For this review, take the finished solid that the model builds, in its own axes (mm). Face numbers are marked on the shaded views. Round coordinates to 2 decimals unless told otherwise and drop trailing zeros. Write each loop counter-clockwise with the first axis right and the second up, starting at its lowest first coordinate (ties: lowest second). Pieces come first, ordered by that corner, then holes. Notation, with made-up numbers: (83.5, -14.5) -> (95.5, -14.5) arc R19 cw to (95.5, -2.5) -> close; hole circle Ø8 at (61, 13). An arc over 180 degrees is marked (long way). Write item = value, one per line. Start each with the question number.
```python
from build123d import *

# Parameters (mm, degrees)
F0_R     = 16.5
F0_R_2   = 14
F1_DEPTH = 125
F0_R_3   = 19
F2_DEPTH = 65
F3_DEPTH = 60
F4_SIZE  = 2.49999


# Not quite as in the source:
# - a fillet or chamfer is up to 0.001 mm smaller than in the source, because OpenCascade refuses the exact size


with BuildPart() as f1:
    # F0 (on Top) → F1 (new body)
    with BuildSketch(Plane.XY):
        Circle(F0_R)
        Circle(F0_R_2, mode=Mode.SUBTRACT)
    extrude(amount=F1_DEPTH)

    # F0 (on Top) → F2 (join)
    with BuildSketch(Plane.XY):
        Circle(F0_R_3)
        Circle(F0_R, mode=Mode.SUBTRACT)
    extrude(amount=F2_DEPTH)

    # F0 (on Top) → F3 (cut)
    with BuildSketch(Plane.XY):
        Circle(F0_R_3)
        Circle(F0_R, mode=Mode.SUBTRACT)
    extrude(amount=F3_DEPTH, mode=Mode.SUBTRACT)

    # F4 (size 2.5 in the source; OpenCascade refuses exactly that, so slightly less here)
    f4_edges = [f1.edges().sort_by_distance(p)[0] for p in [
        (-16.5, 0, 60),
        (-16.5, 0, 65),
    ]]
    chamfer(f4_edges, length=F4_SIZE)


solid = f1.part
```
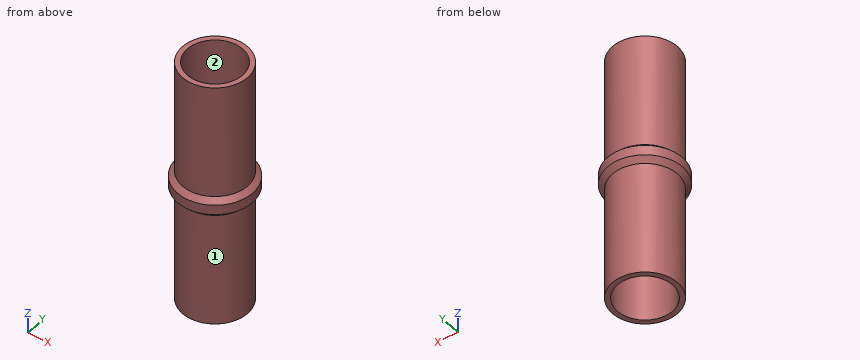
1. Consider section C-C, the plane z = 54.5. Give the boundary of the cut face in (x, y).
2. Wall thickness on L1, parallel to Y at x = 0, z = 27; L2, parallel to X at y = 10, z = 78.5; L3, parallel to Y at x = 8.5, z = 65: over which ranges is each line inside the solid? List them lowest first. Write a range as from..to.
3. Draft analysis for pull direction Y (two halves, no side actions). For the marked faces 1 and 2, state which applies: +Y half, -Y half, draft (parallel to the pull), parting line (faces both ways), or undercut.
4. Clearance check with flat-ended pins moving along their axes: pin 1 Ø12 at (x, z) = (-8, 83) entering from +Y; pin 2 Ø8 at (y, z) = (6, 84.5) entering from -X; pin 3 Ø1 at (x, z) = (10.5, 79.5) entering from -Y; pin 4 Ø1.5 at (x, y) = (-11, 10) entering from -Z. State where each tip first meets the part, or that it passes through.
Outcome:
q1.outline = circle Ø33 at (0, 0); hole circle Ø28 at (0, 0)
q2.L1 = -16.5..-14, 14..16.5
q2.L2 = -13.12..-9.8, 9.8..13.12
q2.L3 = -16.99..-11.12, 11.12..16.99
q3.face_1 = parting line
q3.face_2 = undercut
q4.pin_1 = 16.38
q4.pin_2 = -16.38
q4.pin_3 = -13.12
q4.pin_4 = 0
